Verification items for this drawing (mm, ordinates from the low corner). A direction names the side the tool comes from. Give positions to 0.01 mm unless a question says otherwise; leave off trailing zeros. Order: outer loops, then holes, each group sorted by start corner. A loop starts at its lowest first (then second) coordinate and runs counter-clockwise, first axis right, second up. Notation, with made-up numbers: M -22,56 L -1,56 A9 cw -1,65 Z; hole C 0,34.25 d2. An arc over 180 degrees is marked long. Answer as a JSON object with one key per item and string values.
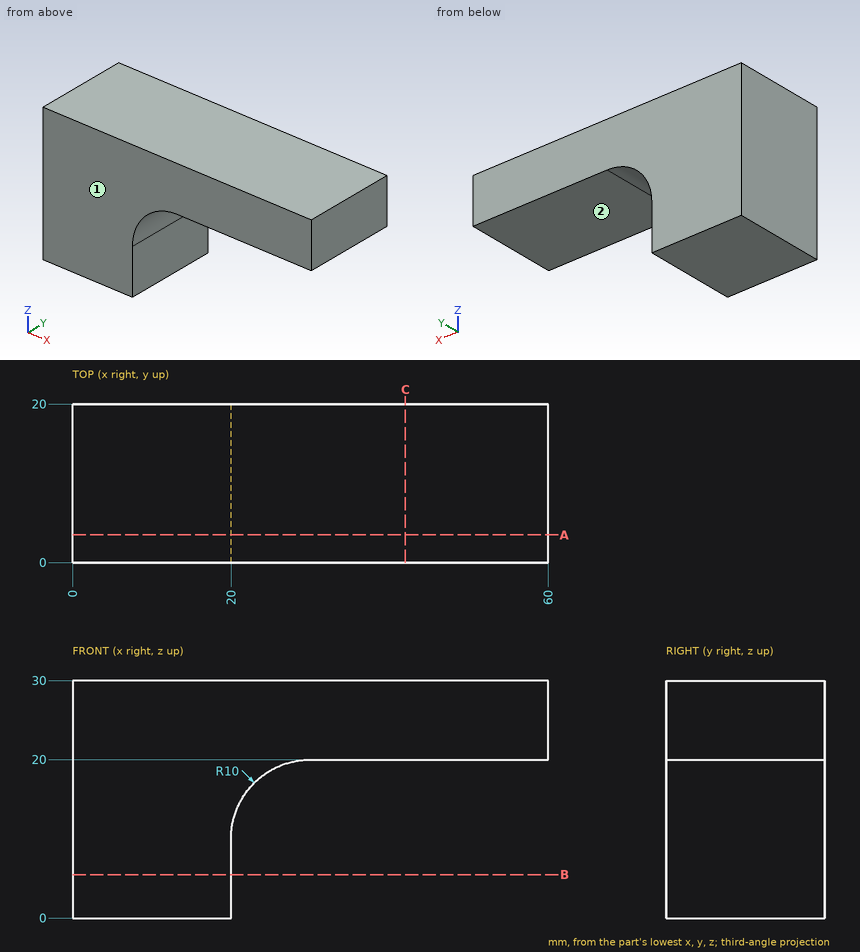
Q1. Section check A-A on y = 3.5. Record the cut outline in (x, z).
Resolved:
{"outline": "M 0,0 L 20,0 L 20,10 A10 cw 30,20 L 60,20 L 60,30 L 0,30 Z"}
Q2. Section check C-C on x = 42. Record the cut outline in (y, z).
Resolved:
{"outline": "M 0,20 L 20,20 L 20,30 L 0,30 Z"}
Q3. Gauge pin test, flat ends, axial feed: pin 1 Ø12 at (x, y) = (33, 4.5) entering from -Z; pin 2 Ø5 at (y, z) = (12, 6.5) entering from +X. Record the tip position at first contact, or that the pin passes through.
Resolved:
{"pin 1": "stops at z = 19.54", "pin 2": "stops at x = 20"}
Q4. Tool access check on the marked faces 1 and 2. Record the directions out of +Z, -Z, +X, -X, +Y, -Y that give a thin tool (end or side, any length) a straight path to the whole face; none if there is none.
Resolved:
{"face 1": "+Z, -Z, +X, -X, -Y", "face 2": "-Z, +X, +Y, -Y"}
Q5. Material ranges on L1, parallel to X at y = 4.75, z = 5.5; L2, parallel to Z at x = 32, y = 14.25; L3, parallel to X at y = 11, z = 19, recorded low to high.
Resolved:
{"L1": "x = 0 to 20", "L2": "z = 20 to 30", "L3": "x = 0 to 25.64"}
Q6. Section check B-B on z = 5.5. Record the cut outline in (x, y).
Resolved:
{"outline": "M 0,0 L 20,0 L 20,20 L 0,20 Z"}
